from build123d import *

# Parameters (mm, degrees)
EXTRUDE_1_DEPTH     = 4
SKETCH_2_R          = 1.4
EXTRUDE_2_DEPTH     = 3.5
CUT_EXTRUDE_1_DEPTH = 2.5
SKETCH_6_R          = 1.8
CUT_EXTRUDE_2_DEPTH = 8.5
SKETCH_7_R          = 1.8
EXTRUDE_3_DEPTH     = 5


with BuildPart() as part:
    # ｽｹｯﾁ1 → ﾎﾞｽ - 押し出し1 (new body)
    with BuildSketch(Plane.XY):
        with BuildLine():
            Line((-6.75, 2.453738644), (-8.915063509, 1.203738644))
            Line((-8.915063509, 1.203738644), (-10.537880917, 2.705877559))
            ThreePointArc((-10.537880917, 2.705877559), (-11.098076211, 6.407477288), (-7.612299165, 7.773133797))
            Line((-7.612299165, 7.773133797), (-5.5, 7.118802154))
            Line((-5.5, 7.118802154), (-5.5, 4.618802154))
            Line((-5.5, 4.618802154), (5.5, 4.618802154))
            Line((5.5, 4.618802154), (5.5, 7.118802154))
            Line((5.5, 7.118802154), (7.612299165, 7.773133797))
            ThreePointArc((7.612299165, 7.773133797), (11.098076211, 6.407477288), (10.537880917, 2.705877559))
            Line((10.537880917, 2.705877559), (8.915063509, 1.203738644))
            Line((8.915063509, 1.203738644), (6.75, 2.453738644))
            Line((6.75, 2.453738644), (1.25, -7.072540798))
            Line((1.25, -7.072540798), (3.415063509, -8.322540798))
            Line((3.415063509, -8.322540798), (2.925581753, -10.479011356))
            ThreePointArc((2.925581753, -10.479011356), (0, -12.814954576), (-2.925581753, -10.479011356))
            Line((-2.925581753, -10.479011356), (-3.415063509, -8.322540798))
            Line((-3.415063509, -8.322540798), (-1.25, -7.072540798))
            Line((-1.25, -7.072540798), (-6.75, 2.453738644))
        make_face()
    extrude(amount=EXTRUDE_1_DEPTH)

    # ｽｹｯﾁ2 → ﾎﾞｽ - 押し出し2 (add)
    with BuildSketch(Plane.XY.offset(4)):
        with Locations((-8.5, 4.907477288)):
            Circle(SKETCH_2_R)
        with Locations((0, -9.814954576)):
            Circle(SKETCH_2_R)
        with Locations((8.5, 4.907477288)):
            Circle(SKETCH_2_R)
    extrude(amount=EXTRUDE_2_DEPTH)

    # ｽｹｯﾁ4 → ｶｯﾄ - 押し出し1 (cut)
    with BuildSketch(Plane.XY.offset(4)):
        Polygon((-1.674315781, -2.9), (1.674315781, -2.9), (3.348631561, 0), (1.674315781, 2.9), (-1.674315781, 2.9), (-3.348631561, 0), align=None)
    extrude(amount=-CUT_EXTRUDE_1_DEPTH, mode=Mode.SUBTRACT)

    # ｽｹｯﾁ6 → ｶｯﾄ - 押し出し2 (cut, through all)
    with BuildSketch(Plane(origin=(0, 0, 0), x_dir=(-1, 0, 0), z_dir=(0, 0, -1))):
        Circle(SKETCH_6_R)
    extrude(amount=-CUT_EXTRUDE_2_DEPTH, mode=Mode.SUBTRACT)

    # ｽｹｯﾁ7 → ﾎﾞｽ - 押し出し3 (add)
    with BuildSketch(Plane(origin=(0, 0, 0), x_dir=(-1, 0, 0), z_dir=(0, 0, -1))):
        with BuildLine():
            Line((-8.915063509, 1.203738644), (-6.75, 2.453738644))
            Line((-6.75, 2.453738644), (-1.25, -7.072540798))
            Line((-1.25, -7.072540798), (-3.415063509, -8.322540798))
            Line((-3.415063509, -8.322540798), (-2.925581753, -10.479011356))
            ThreePointArc((-2.925581753, -10.479011356), (0, -12.814954576), (2.925581753, -10.479011356))
            Line((2.925581753, -10.479011356), (3.415063509, -8.322540798))
            Line((3.415063509, -8.322540798), (1.25, -7.072540798))
            Line((1.25, -7.072540798), (6.75, 2.453738644))
            Line((6.75, 2.453738644), (8.915063509, 1.203738644))
            Line((8.915063509, 1.203738644), (10.537880917, 2.705877559))
            ThreePointArc((10.537880917, 2.705877559), (11.098076211, 6.407477288), (7.612299165, 7.773133797))
            Line((7.612299165, 7.773133797), (5.5, 7.118802154))
            Line((5.5, 7.118802154), (5.5, 4.618802154))
            Line((5.5, 4.618802154), (-5.5, 4.618802154))
            Line((-5.5, 4.618802154), (-5.5, 7.118802154))
            Line((-5.5, 7.118802154), (-7.612299165, 7.773133797))
            ThreePointArc((-7.612299165, 7.773133797), (-11.098076211, 6.407477288), (-10.537880917, 2.705877559))
            Line((-10.537880917, 2.705877559), (-8.915063509, 1.203738644))
        make_face()
        Circle(SKETCH_7_R, mode=Mode.SUBTRACT)
    extrude(amount=EXTRUDE_3_DEPTH)


solid = part.part
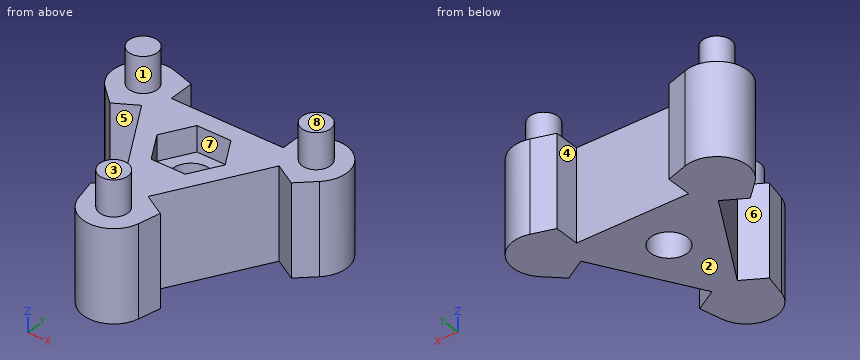
Check sheet for the modelled part. Datum: model origin and axes. Units: mm. Face numbers are marked on the shaded views. A direction names the side the tool comes from. Round coordinates to 2 decimals unless told otherwise and drop trailing zeros. Loops run counter-clockwise (first coordinate to the right, second up) from the corner with the lowest first, then second, coordinate; pieces in that order, holes last.
1. Gauge pin test, flat ends, axial feed: pin 1 Ø1 at (y, z) = (-0.5, -3.5) entering from -X; pin 2 Ø1.2 at (x, z) = (0, 3) entering from +Y; pin 3 Ø1.5 at (y, z) = (-5, 2.5) entering from +X; pin 4 Ø1 at (y, z) = (2.5, 6) entering from -X. Record the tip position at first contact, or that the pin passes through.
2. Scan lines: probe 1 along X at (y, z) = (1.5, -0.25); probe 2 along Z at (x, y) = (2.5, -2.25); probe 3 along X at (y, z) = (0.25, -2.5). Record each from-to range of solid material in increasing order.
3. Sectioned sample at B-B on x = 0. Record the boundary of the cut face in (y, z), and give its area (3 significant figures).
4. Mould release check, pull along X, two halves, no side actions. Record for the marked faces 6, 7 and 8: released by +X, released by -X, zero draft, split by the parting line, or undercut.
5. Sectioned sample at C-C on x = 8.5. Record the boundary of the cut face in (y, z).
6. Set-up check for the marked faces 1, 2, 3, 4 and 5: record each of +Z, -Z, +X, -X, +Y, -Y from which the full face is reachable in a straight line by a thin tool's end or side.
7. Sectioned sample at A-A on z = 0.75. Record the boundary of the cut face in (x, y).
8. Sectioned sample at D-D on y = -6. Record the boundary of the cut face in (x, z), and give its area (3 significant figures).
Recorded:
1. pin 1: stops at x = -5.33
1. pin 2: stops at y = 4.62
1. pin 3: stops at x = 2.88
1. pin 4: passes through
2. probe 1: x = -9.24 to -8.4, -6.2 to -0.99, 0.99 to 6.2, 8.4 to 9.24
2. probe 2: z = -5 to 4
2. probe 3: x = -5.48 to -1.78, 1.78 to 5.48
3. outline: (-12.81, -5) - (-1.8, -5) - (-1.8, 1.5) - (-2.9, 1.5) - (-2.9, 4) - (-8.41, 4) - (-8.41, 7.5) - (-11.21, 7.5) - (-11.21, 4) - (-12.81, 4) - close; (1.8, -5) - (4.62, -5) - (4.62, 4) - (2.9, 4) - (2.9, 1.5) - (1.8, 1.5) - close
3. area: 129 mm2
4. face 6: released by -X
4. face 7: undercut
4. face 8: zero draft
5. outline: (1.44, -5) - (7.91, -5) - (7.91, 4) - (6.31, 4) - (6.31, 7.5) - (3.51, 7.5) - (3.51, 4) - (1.44, 4) - close
6. face 1: +Z
6. face 2: -Z, +X, -X, +Y, -Y
6. face 3: +Z, +X, -X, +Y, -Y
6. face 4: +Z, -Z, +Y
6. face 5: +Z, -Z, -Y
7. outline: (-10.54, 2.71) - (-8.92, 1.2) - (-6.75, 2.45) - (-1.25, -7.07) - (-3.42, -8.32) - (-2.93, -10.48) arc R3 ccw to (2.93, -10.48) - (3.42, -8.32) - (1.25, -7.07) - (6.75, 2.45) - (8.92, 1.2) - (10.54, 2.71) arc R3 ccw to (7.61, 7.77) - (5.5, 7.12) - (5.5, 4.62) - (-5.5, 4.62) - (-5.5, 7.12) - (-7.61, 7.77) arc R3 ccw to start; hole circle Ø3.6 at (0, 0)
8. outline: (-1.87, -5) - (1.87, -5) - (1.87, 4) - (-1.87, 4) - close
8. area: 33.6 mm2
